Could you check a few things on this model? Use its own coordinates, in mm. A direction names the side the tool comes from. Give positions to 0.01 mm unless a question says otherwise; leave off trailing zeros. Order: outer loops, then holes, each group sorted by start corner. A loop starts at its lowest first (then second) coordinate and runs counter-clockwise, first axis right, second up.
(1) Imagine slicing it at B-B, the plane y = 50. Write out the boundary of the cut face in (x, z), then the cut area to 3 significant figures.
(2) Imagine slicing it at A-A, the plane x = 261. Write out the boundary of the cut face in (y, z), then the cut area to 3 significant figures.
(3) Imagine slicing it at C-C, the plane z = -7.25. Write out the boundary of the cut face in (x, y), then the cut area to 3 significant figures.
(4) If I drill on probe 1 along X at (y, z) = (52, -10.25); probe 2 along Y at (x, z) = (260.5, -16.5); probe 3 along Z at (x, y) = (240, 52.5), over which ranges is the centre line in solid material (lowest first)?
(5) On a 3-axis mill with a long thin cutter (end or side, diameter ignored), from which of +Z, -Z, +X, -X, +Y, -Y can I reach the whole of each face in a straight line? I mean faces 1 (the flat face through (261, 65.75, -13)), 2 (the flat face through (245.25, 50, -13)), 3 (the flat face through (272, 29.7, -2)), 4 (the flat face through (276.75, 50, -13)). Say none if no direction works.
(6) Imagine slicing it at D-D, the plane y = 68.5. Write out the boundary of the cut face in (x, z), then the cut area to 3 significant figures.
(7) Will these pins go through, and if not, where does the flat tip stop? pin 1 (5 mm diameter, centred on x = 252.5, z = -9, fed in from +Y); pin 2 (4 mm diameter, centred on y = 51, z = -6, fed in from +X); pin 3 (10.5 mm diameter, centred on y = 46, z = -11, fed in from -X).
from build123d import *

# Parameters (mm, degrees)
SKETCH045_R  = 25
PAD017_DEPTH = 2.5
SKETCH046_R  = 22.75
PAD018_DEPTH = 6
SKETCH047_W  = 31.5
SKETCH047_H  = 31.5
PAD019_DEPTH = 9.5


with BuildPart() as part:
    # Sketch045 → Pad017 (new body)
    with BuildSketch(Plane.XY):
        Circle(SKETCH045_R)
    extrude(amount=PAD017_DEPTH)

    # Sketch046 (on Face2 of Pad017) → Pad018 (join)
    with BuildSketch(Plane(origin=(0, 0, 0), x_dir=(1, 0, 0), z_dir=(0, 0, -1))):
        Circle(SKETCH046_R)
    extrude(amount=PAD018_DEPTH)

    # Sketch047 (on Face5 of Pad018) → Pad019 (join)
    with BuildSketch(Plane(origin=(0, 0, -6), x_dir=(1, 0, 0), z_dir=(0, 0, -1))):
        Rectangle(SKETCH047_W, SKETCH047_H)
    extrude(amount=PAD019_DEPTH)


with BuildPart() as part_1:
    # Body009 placement: moved
    add(part.part.moved(Location((261, 50, -2))))


solid = part_1.part
Answer block:
1. outline: (236, -2) - (238.25, -2) - (238.25, -8) - (245.25, -8) - (245.25, -17.5) - (276.75, -17.5) - (276.75, -8) - (283.75, -8) - (283.75, -2) - (286, -2) - (286, 0.5) - (236, 0.5) - close
1. area: 697 mm2
2. outline: (25, -2) - (27.25, -2) - (27.25, -8) - (34.25, -8) - (34.25, -17.5) - (65.75, -17.5) - (65.75, -8) - (72.75, -8) - (72.75, -2) - (75, -2) - (75, 0.5) - (25, 0.5) - close
2. area: 697 mm2
3. outline: circle Ø45.5 at (261, 50)
3. area: 1,630 mm2
4. probe 1: x = 245.25 to 276.75
4. probe 2: y = 34.25 to 65.75
4. probe 3: z = -8 to 0.5
5. face 1: -Z, +X, -X, +Y
5. face 2: -Z, -X, +Y, -Y
5. face 3: -Z
5. face 4: -Z, +X, +Y, -Y
6. outline: (244.18, -2) - (247.76, -2) - (247.76, -8) - (274.24, -8) - (274.24, -2) - (277.82, -2) - (277.82, 0.5) - (244.18, 0.5) - close
6. area: 243 mm2
7. pin 1: stops at y = 71.89
7. pin 2: stops at x = 283.75
7. pin 3: stops at x = 238.25
